Input: part model. Units: mm. Frame: model coordinates. Face numbers are marked on the shaded views. A direction names the side the tool comes from. Round coordinates to 2 decimals unless told otherwise and drop trailing zeros. Loops run counter-clockwise (first coordinate to the right, second up) from the corner with the lowest first, then second, coordinate; pieces in that order, holes last.
(1) First-contact query: pin 1 Ø2.5 at (y, z) = (16, 5) entering from +X; pin 2 Ø3 at (y, z) = (-6, 4) entering from +X; pin 3 Ø2 at (x, z) = (3, 3.5) entering from +Y; pin 4 Ø4 at (y, z) = (18, 4) entering from -X. Flat tips, straight axial feed; report the tip coordinate or a pass-through.
(2) Access query for the marked faces 1, 2 and 3. Directions: +Z, -Z, +X, -X, +Y, -Y. A direction counts if a zero-diameter tool reaches every point of the face in a straight line with its end or side. Return the directions, or none.
(3) Draft query along X for the marked faces 4, 5, 6 and 7. Return one class per face: released by +X, released by -X, zero draft, split by the parting line, or undercut.
(4) Cut plane A-A, the plane y = -6. Output: boundary loops of the cut face in (x, z), and give its area (3 significant figures).
(5) Cut plane C-C, the plane y = 1.5. Output: boundary loops of the cut face in (x, z).
(6) Cut plane D-D, the plane z = 1. Output: boundary loops of the cut face in (x, y).
(7) Line query: line 1 (X direction, y = -3, z = 1); line 2 (X direction, y = 15, z = 5); line 3 (Z direction, x = 11.3, y = 18). Output: solid intervals per line, ascending.
(8) Cut plane B-B, the plane x = 13. Output: boundary loops of the cut face in (y, z), and give its area (3 significant figures).
from build123d import *

# Parameters (mm, degrees)
F1_DEPTH      = 8
F2_W          = 19.5
F2_H          = 12
F2_W_2        = 23
F3_DEPTH      = 8
F4_R          = 1.6
F5_DEPTH      = 32
F6_R          = 1.6
F7_DEPTH      = 28
F8_SIZE       = 2
F10_DEPTH     = 9.751
F11_T1_DEPTH  = 14.7867319519
F11_T3_DEPTH  = 14.7867319519
F11_T5_DEPTH  = 14.5367319519
F11_T7_DEPTH  = 14.5367319519
F11_T12_DEPTH = 25.7867319519
F11_T18_DEPTH = 29.2867319519
F11_T24_ANGLE = 117.8974179381
F11_T30_ANGLE = 101.5178089871


# Not quite as in the source:
# - a fillet or chamfer that OpenCascade refuses, or shapes differently, is made with other operations: its cross-section is extruded or revolved along the edge and cut away or added


with BuildPart() as f1:
    # F0 (on Top) → F1 (new body)
    with BuildSketch(Plane.XY):
        Polygon((14, 22), (-14, 22), (-14, 12), (-16, 0), (-16, -10), (16, -10), (16, 0), (14, 12), align=None)
    extrude(amount=F1_DEPTH)

    # F2 (on face) → F3 (cut, through all)
    with BuildSketch(Plane.XY.offset(8)):
        with Locations((0, 16)):
            Rectangle(F2_W, F2_H)
        with Locations((0, -4)):
            Rectangle(F2_W_2, F2_H)
    extrude(amount=-F3_DEPTH, mode=Mode.SUBTRACT)

    # F4 (on face) → F5 (cut, through all)
    with BuildSketch(Plane.YZ.offset(16)):
        with Locations((-6, 4)):
            Circle(F4_R)
    extrude(amount=-F5_DEPTH, mode=Mode.SUBTRACT)

    # F6 (on face) → F7 (cut, through all)
    with BuildSketch(Plane.YZ.offset(14)):
        with Locations((18, 4)):
            Circle(F6_R)
    extrude(amount=-F7_DEPTH, mode=Mode.SUBTRACT)

    # F8
    f8_edges = [f1.edges().sort_by_distance(p)[0] for p in [
        (9.75, 10, 4),
        (-9.75, 10, 4),
        (11.5, 2, 4),
        (-11.5, 2, 4),
    ]]
    chamfer(f8_edges, length=F8_SIZE)

    # F9 (on face) → F10 (cut, through all)
    with BuildSketch(Plane.XZ.offset(-2)):
        with BuildLine():
            Line((9.5, 8), (-9.5, 8))
            ThreePointArc((-9.5, 8), (0, 4.6081867662), (9.5, 8))
        make_face()
    extrude(amount=-F10_DEPTH, mode=Mode.SUBTRACT)

    # F11: chamfer of 2 on 12 edges, made by hand

    # F11_s2 → F11_t1 (cut)
    with BuildSketch(Plane.YZ.offset(-21.1433659759)):
        Polygon((-10, 6), (-8, 8), (-10, 8), align=None)
        Polygon((-8, 0), (-10, 2), (-10, 0), align=None)
    extrude(amount=F11_T1_DEPTH, mode=Mode.SUBTRACT)

    # F11_s4 → F11_t3 (cut)
    with BuildSketch(Plane.YZ.offset(6.3566340241)):
        Polygon((-10, 6), (-8, 8), (-10, 8), align=None)
        Polygon((-8, 0), (-10, 2), (-10, 0), align=None)
    extrude(amount=F11_T3_DEPTH, mode=Mode.SUBTRACT)

    # F11_s6 → F11_t5 (cut)
    with BuildSketch(Plane.YZ.offset(4.6066340241)):
        Polygon((22, 6), (20, 8), (22, 8), align=None)
        Polygon((20, 0), (22, 2), (22, 0), align=None)
    extrude(amount=F11_T5_DEPTH, mode=Mode.SUBTRACT)

    # F11_s8 → F11_t7 (cut)
    with BuildSketch(Plane.YZ.offset(-19.1433659759)):
        Polygon((20, 0), (22, 2), (22, 0), align=None)
        Polygon((22, 6), (20, 8), (22, 8), align=None)
    extrude(amount=F11_T7_DEPTH, mode=Mode.SUBTRACT)


with BuildPart() as f11_tool10:
    # F11_s11 → F11_t12 (new body)
    with BuildSketch(Plane.YZ.offset(-12.8933659759)):
        Polygon((8, 0), (10, 2), (10, 0), align=None)
    extrude(amount=F11_T12_DEPTH)

    split(bisect_by=Plane(origin=(-1.125, 1.125, 0), x_dir=(0, 0, 1), z_dir=(-0.7071067812, 0.7071067812, 0)), keep=Keep.TOP)

    split(bisect_by=Plane(origin=(1.125, 1.125, 0), x_dir=(0, 0, 1), z_dir=(0.7071067812, 0.7071067812, 0)), keep=Keep.TOP)


with BuildPart() as f1_1:
    add(f1.part)

    # F11_t9: cut F11_tool10
    add(f11_tool10.part, mode=Mode.SUBTRACT)


with BuildPart() as f11_tool16:
    # F11_s17 → F11_t18 (new body)
    with BuildSketch(Plane.YZ.offset(14.6433659759)):
        Polygon((4, 0), (2, 2), (2, 0), align=None)
    extrude(amount=-F11_T18_DEPTH)

    split(bisect_by=Plane(origin=(5.75, 5.75, 0), x_dir=(0, 0, 1), z_dir=(-0.7071067812, -0.7071067812, 0)), keep=Keep.TOP)

    split(bisect_by=Plane(origin=(-5.75, 5.75, 0), x_dir=(0, 0, 1), z_dir=(0.7071067812, -0.7071067812, 0)), keep=Keep.TOP)


with BuildPart() as f1_2:
    add(f1_1.part)

    # F11_t15: cut F11_tool16
    add(f11_tool16.part, mode=Mode.SUBTRACT)


with BuildPart() as f11_tool22:
    # F11_s23 → F11_t24 (revolve)
    with BuildSketch(Plane(origin=(-8.664727501, 0, 14.3913305034), x_dir=(0, 1, 0), z_dir=(-0.5158052023, 0, 0.8567058966))):
        Polygon((2, 6.8859952574), (4, 4.8859952574), (2, 4.8859952574), align=None)
    revolve(axis=Axis((0, 2, 19.6081867662), (0, -1, 0)), revolution_arc=F11_T24_ANGLE)

    split(bisect_by=Plane(origin=(5.75, 5.75, 0), x_dir=(0, 0, 1), z_dir=(-0.7071067812, -0.7071067812, 0)), keep=Keep.TOP)

    split(bisect_by=Plane(origin=(-5.75, 5.75, 0), x_dir=(0, 0, 1), z_dir=(0.7071067812, -0.7071067812, 0)), keep=Keep.TOP)


with BuildPart() as f1_3:
    add(f1_2.part)

    # F11_t21: cut F11_tool22
    add(f11_tool22.part, mode=Mode.SUBTRACT)


with BuildPart() as f11_tool28:
    # F11_s29 → F11_t30 (revolve)
    with BuildSketch(Plane(origin=(-9.6066653022, 0, 11.7617013204), x_dir=(0, 1, 0), z_dir=(-0.6325849704, 0, 0.7744909652))):
        Polygon((10, 4.596155754), (8, 2.596155754), (10, 2.596155754), align=None)
    revolve(axis=Axis((0, 10, 19.6081867662), (0, -1, 0)), revolution_arc=F11_T30_ANGLE)

    split(bisect_by=Plane(origin=(-1.125, 1.125, 0), x_dir=(0, 0, 1), z_dir=(-0.7071067812, 0.7071067812, 0)), keep=Keep.TOP)

    split(bisect_by=Plane(origin=(1.125, 1.125, 0), x_dir=(0, 0, 1), z_dir=(0.7071067812, 0.7071067812, 0)), keep=Keep.TOP)


with BuildPart() as f1_4:
    add(f1_3.part)

    # F11_t27: cut F11_tool28
    add(f11_tool28.part, mode=Mode.SUBTRACT)


solid = f1_4.part
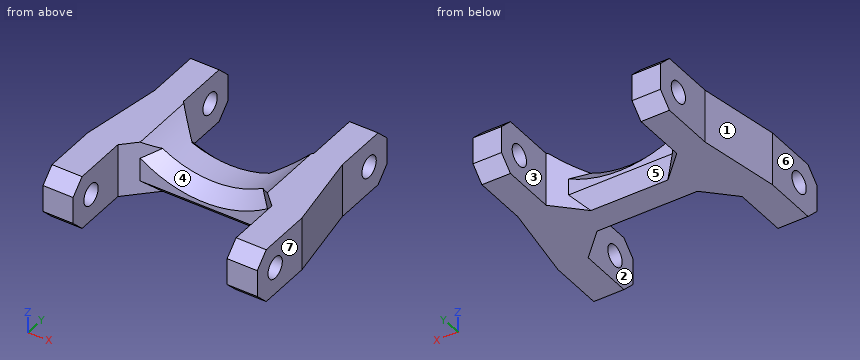
Reported:
1. pin 1: stops at x = 14
1. pin 2: passes through
1. pin 3: stops at y = 10
1. pin 4: stops at x = -14
2. face 1: +Z, -Z, -X, +Y
2. face 2: +Z, -Z, -Y
2. face 3: +Z, -Z, +Y
3. face 4: undercut
3. face 5: undercut
3. face 6: released by -X
3. face 7: released by +X
4. outline: (-16, 0) - (-11.5, 0) - (-11.5, 2.4) - (-16, 2.4) - close; (-16, 5.6) - (-11.5, 5.6) - (-11.5, 8) - (-16, 8) - close; (11.5, 0) - (16, 0) - (16, 2.4) - (11.5, 2.4) - close; (11.5, 5.6) - (16, 5.6) - (16, 8) - (11.5, 8) - close
4. area: 43.2 mm2
5. outline: (-15.75, 0) - (-10, 0) - (-10, 8) - (-15.75, 8) - close; (10, 0) - (15.75, 0) - (15.75, 8) - (10, 8) - close
6. outline: (-16, -9) - (-11.5, -9) - (-11.5, 0) - (-8.5, 3) - (8.5, 3) - (11.5, 0) - (11.5, -9) - (16, -9) - (16, 0) - (14, 12) - (14, 21) - (9.75, 21) - (9.75, 12) - (6.75, 9) - (-6.75, 9) - (-9.75, 12) - (-9.75, 21) - (-14, 21) - (-14, 12) - (-16, 0) - close
7. line 1: x = -16 to -11.5, 11.5 to 16
7. line 2: x = -14 to -9.75, 9.75 to 14
7. line 3: z = 0 to 2.4, 5.6 to 8
8. outline: (-10, 2) - (-8, 0) - (20, 0) - (22, 2) - (22, 6) - (20, 8) - (-8, 8) - (-10, 6) - close; hole circle Ø3.2 at (-6, 4); hole circle Ø3.2 at (18, 4)
8. area: 232 mm2
